from build123d import *

# Parameters (mm, degrees)
F0_R     = 56.02
F0_R_2   = 10
F1_DEPTH = 28
F2_R     = 37.5
F2_R_2   = 10
F3_DEPTH = 6
F4_R     = 45
F4_R_2   = 10
F5_DEPTH = 18
F6_R     = 18
F6_R_2   = 10
F7_DEPTH = 9
F9_DEPTH = 25


with BuildPart() as f1:
    # F0 (on Top) → F1 (new body)
    with BuildSketch(Plane.XY):
        Circle(F0_R)
        Circle(F0_R_2, mode=Mode.SUBTRACT)
    extrude(amount=F1_DEPTH)

    # F2 (on face) → F3 (join)
    with BuildSketch(Plane.XY.offset(28)):
        Circle(F2_R)
        Circle(F2_R_2, mode=Mode.SUBTRACT)
    extrude(amount=F3_DEPTH)

    # F4 (on face) → F5 (cut)
    with BuildSketch(Plane(origin=(0, 0, 0), x_dir=(1, 0, 0), z_dir=(0, 0, -1))):
        Circle(F4_R)
        Circle(F4_R_2, mode=Mode.SUBTRACT)
    extrude(amount=-F5_DEPTH, mode=Mode.SUBTRACT)

    # F6 (on face) → F7 (join)
    with BuildSketch(Plane(origin=(0, 0, 18), x_dir=(1, 0, 0), z_dir=(0, 0, -1))):
        Circle(F6_R)
        Circle(F6_R_2, mode=Mode.SUBTRACT)
    extrude(amount=F7_DEPTH)

    # F8 (on face) → F9 (cut)
    with BuildSketch(Plane.XY.offset(34)):
        with BuildLine():
            ThreePointArc((3, -9.5393920142), (0, -10), (-3, -9.5393920142))
            Line((-3, -9.5393920142), (-3, -13.0393920142))
            Line((-3, -13.0393920142), (3, -13.0393920142))
            Line((3, -13.0393920142), (3, -9.5393920142))
        make_face()
    extrude(amount=-F9_DEPTH, mode=Mode.SUBTRACT)


solid = f1.part
The model under review builds one solid part; all positions refer to its coordinate system, in mm. A direction names the side the tool comes from. Give positions to 0.01 mm unless a question says otherwise; leave off trailing zeros. Write each loop counter-clockwise with the first axis right and the second up, starting at its lowest first coordinate (ties: lowest second). Pieces come first, ordered by that corner, then holes.
1. For P1, Ø12, axis at x = -38, y = -33.5, coming from the +Z side; P2, Ø4, axis at y = -12, z = 25, coming from the -X side; P3, Ø1.8, axis at y = -11.5, z = 23.5, coming from the +X side; P4, Ø1, axis at y = -41, z = 29.5, coming from the +X side, all flat-tipped, find the tip position at first contact; note any pin that passes through.
2. Wall thickness on L1, parallel to Y at x = 0, z = 17.25; L2, parallel to Z at x = -24.5, y = 6; L3, parallel to Z at x = -36.5, y = -32.5: over which ranges is each line inside the solid? List them lowest first.
3. Add section C-C, the plane x = 0. Write out the cut boundary in (y, z).
4. Add section B-B, the plane y = 0. Write out the cut boundary in (x, z), plus the area to 3 significant figures.
5. Draft analysis for pull direction X (two halves, no side actions). For faces 5 (the flat face through (-3, -11, 22)), 6 (the cylindrical face through (-2.343, -17.847, 13.563)), 7 (the cylindrical face through (-4.88, 37.18, 30.96)), 8 (the flat face through (0, 46, 0)), state which applies: +X half, -X half, draft (parallel to the pull), parting line (faces both ways), or undercut.
6. Add section D-D, the plane z = 21. Write out the cut boundary in (x, y), plus the area to 3 significant figures.
7. Add section A-A, the plane z = 13. Write out the cut boundary in (x, y).
8. Tool access review of faces 1 (the flat face through (19, -1, 18)), 2 (the flat face through (12, -37, 28)), 3 (the flat face through (0, -13.039, 22)), 4 (the flat face through (8, -8, 34)): name each direction out of +Z, -Z, +X, -X, +Y, -Y from which nothing blocks a thin tool from reaching the whole face with its end or side.
Worked answers:
1. P1: stops at z = 28
1. P2: stops at x = -55.12
1. P3: stops at x = 55.01
1. P4: passes through
2. L1: y = -56.02 to -45, -18 to -13.04, 10 to 18, 45 to 56.02
2. L2: z = 18 to 34
2. L3: z = 0 to 28
3. outline: (-56.02, 0) - (-45, 0) - (-45, 18) - (-18, 18) - (-18, 9) - (-13.04, 9) - (-13.04, 34) - (-37.5, 34) - (-37.5, 28) - (-56.02, 28) - close; (10, 9) - (18, 9) - (18, 18) - (45, 18) - (45, 0) - (56.02, 0) - (56.02, 28) - (37.5, 28) - (37.5, 34) - (10, 34) - close
4. outline: (-56.02, 0) - (-45, 0) - (-45, 18) - (-18, 18) - (-18, 9) - (-10, 9) - (-10, 34) - (-37.5, 34) - (-37.5, 28) - (-56.02, 28) - close; (10, 9) - (18, 9) - (18, 18) - (45, 18) - (45, 0) - (56.02, 0) - (56.02, 28) - (37.5, 28) - (37.5, 34) - (10, 34) - close
4. area: 1,790 mm2
5. face 5: undercut
5. face 6: undercut
5. face 7: parting line
5. face 8: draft
6. outline: circle Ø112.04 at (0, 0); hole (-3, -13.04) - (3, -13.04) - (3, -9.54) arc R10 ccw (long way) to (-3, -9.54) - close
6. area: 9,530 mm2
7. outline: circle Ø112.04 at (0, 0); circle Ø36 at (0, 0); hole circle Ø90 at (0, 0); hole (-3, -13.04) - (3, -13.04) - (3, -9.54) arc R10 ccw (long way) to (-3, -9.54) - close
8. face 1: -Z
8. face 2: +Z
8. face 3: +Z, -Z
8. face 4: +Z, +X, -X, +Y, -Y
